Geometry check sheet. Reference: the model listing, model coordinates, mm. Give positions to 0.01 mm unless a question says otherwise; leave off trailing zeros. Order: outer loops, then holes, each group sorted by start corner. A loop starts at its lowest first (then second) coordinate and runs counter-clockwise, first axis right, second up. Notation, with made-up numbers: M 54.25,69.5 L 95.25,69.5 A34 cw 95.25,102.5 Z; hole C 28.5,13.5 d6. An arc over 180 degrees is marked long. Answer as a JSON object with one key per item and string values. Group by question number.
from build123d import *

# Parameters (mm, degrees)
F0_R     = 34.5834158621
F1_DEPTH = 150
F1_TAPER = -5
F2_T     = -2.5
F3_R     = 1


with BuildPart() as f1:
    # F0 (on Top) → F1 (new body)
    with BuildSketch(Plane.XY):
        Circle(F0_R)
    extrude(amount=F1_DEPTH, taper=F1_TAPER)

    # F2
    f2_openings = [f1.faces().sort_by_distance(p)[0] for p in [
        (0, 0, 150),
    ]]
    offset(amount=F2_T, openings=f2_openings, kind=Kind.INTERSECTION)

    # F3
    f3_edges = [f1.edges().sort_by_distance(p)[0] for p in [
        (-47.706715, 0, 150),
        (-45.197166, 0, 150),
    ]]
    fillet(f3_edges, radius=F3_R)


solid = f1.part
1. Release check for a two-part mould opening along Y. For faces 1 (the flat face through (0, 0, 2.5)), 2 (the flat face through (0, 0, 0)), 3 (the conical face through (-41.15, 1.81, 75.5)) record: released by +Y, released by -Y, zero draft, split by the parting line, or undercut.
2. Cross-section at A-A (x = 0). Record the cut outline in (y, z).
3. Thickness scan on line 1 along X through (y, z) = (5, 29.5); line 2 along Z through (x, y) = (14.5, 21); line 3 along Y through (x, z) = (23, 129). Record the ranges inside material, lowest first. Write a range as [from, to].
4. Depth check by flat-ended pin: pin 1 (10 mm diameter, centred on x = -22.5, z = 20.5, fed in from -Y); pin 2 (3 mm diameter, centred on y = 19.5, z = 81.5, fed in from +X); pin 3 (8 mm diameter, centred on y = 30, z = 132.5, fed in from -X). Enter the tip coordinate at first touch or a pass-through.
5. Cross-section at C-C (z = 90.5). Record the cut outline in (x, y), and give its area (3 significant figures).
6. Cross-section at B-B (z = 55.5). Record the cut outline in (x, y).
Report:
{
 "1": {"face 1": "undercut", "face 2": "zero draft", "face 3": "split by the parting line"},
 "2": {"outline": "M -47.61,148.91 L -34.58,0 L 34.58,0 L 47.61,148.91 A1 ccw 46.62,150 L 46.11,150 A1 ccw 45.12,149.09 L 32.29,2.5 L -32.29,2.5 L -45.12,149.09 A1 ccw -46.11,150 L -46.62,150 A1 ccw Z"},
 "3": {"line 1": "x = [-36.83, -34.29], [34.29, 36.83]", "line 2": "z = [0, 2.5]", "line 3": "y = [-39.69, -36.76], [36.76, 39.69]"},
 "4": {"pin 1": "stops at y = -31.94", "pin 2": "stops at x = 37.64", "pin 3": "stops at x = -38.19"},
 "5": {"outline": "C 0,0 d85; hole C 0,0 d79.98", "area": "650 mm2"},
 "6": {"outline": "C 0,0 d78.88; hole C 0,0 d73.86"}
}
